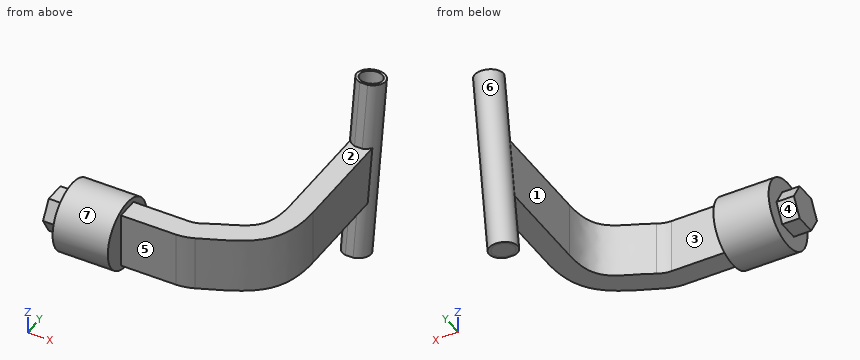
```python
from build123d import *

# Parameters (mm, degrees)
BOSS_EXTRUDE1_DEPTH      = 127
SKETCH2_R                = 78.74
BOSS_EXTRUDE2_DEPTH      = 127
BOSS_EXTRUDE3_DEPTH      = 40.132
BOSS_EXTRUDE4_DEPTH      = 12.7
BOSS_EXTRUDE4_DEPTH_BACK = 63.5
CUT_EXTRUDE4_DEPTH       = 719.599431417
SKETCH7_R                = 25.4
CUT_EXTRUDE5_DEPTH       = 304.8
BOSS_EXTRUDE5_DEPTH      = 50.8
SKETCH9_R                = 25.4
CUT_EXTRUDE6_DEPTH       = 706.793572447
SKETCH10_R               = 28.426883493
BOSS_EXTRUDE6_DEPTH      = 152.4


with BuildPart() as part:
    # Sketch1 → Boss-Extrude1 (new body)
    with BuildSketch(Plane.XY):
        with BuildLine():
            Line((0, 0), (127, 0))
            ThreePointArc((127, 0), (146.783062772, 2.389452828), (165.763803889, 8.456620544))
            add(Edge.make_bspline(
                [(165.763803889, 8.456620544), (215.95075425, 29.910933142), (293.749967936, 60.02479605), (329.40949352, 131.409080947), (329.40949352, 197.581697377)],
                knots=[0, 0, 0, 0, 0.489737158, 1, 1, 1, 1], degree=3))
            Line((329.40949352, 197.581697377), (329.40949352, 431.8))
            Line((329.40949352, 431.8), (278.60949352, 431.8))
            Line((278.60949352, 431.8), (278.60949352, 197.581697377))
            add(Edge.make_bspline(
                [(156.630652755, 58.428868346), (189.028044031, 76.295644753), (253.765909659, 94.018996051), (278.60949352, 141.969854777), (278.60949352, 197.581697377)],
                knots=[0, 0, 0, 0, 0.475110131, 1, 1, 1, 1], degree=3))
            ThreePointArc((156.630652755, 58.428868346), (142.298490244, 52.737817604), (127, 50.8))
            Line((127, 50.8), (0, 50.8))
            Line((0, 50.8), (0, 0))
        make_face()
    extrude(amount=BOSS_EXTRUDE1_DEPTH)

    # Sketch2 → Boss-Extrude2 (add)
    with BuildSketch(Plane.ZY):
        with Locations((63.5, 25.4)):
            Circle(SKETCH2_R)
    extrude(amount=BOSS_EXTRUDE2_DEPTH)

    # Sketch3 → Boss-Extrude3 (add)
    with BuildSketch(Plane.ZY.offset(127)):
        Polygon((63.5, 72.32702988), (22.86, 48.86351494), (22.86, 1.93648506), (63.5, -21.52702988), (104.14, 1.93648506), (104.14, 48.86351494), align=None)
    extrude(amount=BOSS_EXTRUDE3_DEPTH)

    # Sketch4 → Boss-Extrude4 (add, two sides: drawn at the far end of the back side and taken through both)
    with BuildSketch(Plane.ZY.offset(-278.60949352).offset(-BOSS_EXTRUDE4_DEPTH_BACK)):
        Polygon((-123.979561218, 390.165409655), (273.996216856, 449.279655757), (262.901002007, 523.976146929), (-135.074776066, 464.861900827), align=None)
    extrude(amount=BOSS_EXTRUDE4_DEPTH + BOSS_EXTRUDE4_DEPTH_BACK)

    # Sketch6 → Cut-Extrude4 (cut, through all)
    with BuildSketch(Plane(origin=(0, -9.595531889, -64.600151761), x_dir=(-1, 0, 0), z_dir=(0, -0.14692530866024317, -0.9891475894299558))):
        with BuildLine():
            Line((-342.10949352, 404.146909738), (-312.773498747, 404.146909738))
            ThreePointArc((-312.773498747, 404.146909738), (-322.933498747, 460.026909738), (-272.133498747, 434.626909738))
            ThreePointArc((-272.133498747, 434.626909738), (-278.483498747, 415.576909738), (-294.993498747, 404.146909738))
            Line((-294.993498747, 404.146909738), (-265.90949352, 404.146909738))
            Line((-265.90949352, 404.146909738), (-265.90949352, 479.662931787))
            Line((-265.90949352, 479.662931787), (-342.10949352, 479.662931787))
            Line((-342.10949352, 479.662931787), (-342.10949352, 404.146909738))
        make_face()
    extrude(amount=-CUT_EXTRUDE4_DEPTH, mode=Mode.SUBTRACT)

    # Sketch7 → Cut-Extrude5 (cut)
    with BuildSketch(Plane(origin=(0, -9.595531889, -64.600151761), x_dir=(-1, 0, 0), z_dir=(0, -0.14692530866024317, -0.9891475894299558))):
        with Locations(Location((-303.883498747, 434.626909738, 0), (0, 0, 90))):
            Circle(SKETCH7_R)
    extrude(amount=-CUT_EXTRUDE5_DEPTH, mode=Mode.SUBTRACT)

    # Sketch8 → Boss-Extrude5 (add)
    with BuildSketch(Plane.ZY.offset(-278.60949352)):
        Polygon((0, 400.877395826), (0, 426.277395826), (127, 445.141632467), (127, 419.741632467), align=None)
    extrude(amount=-BOSS_EXTRUDE5_DEPTH)

    # Sketch9 → Cut-Extrude6 (cut, through all)
    with BuildSketch(Plane(origin=(0, -9.595531889, -64.600151761), x_dir=(-1, 0, 0), z_dir=(0, -0.14692530866024317, -0.9891475894299558))):
        with Locations(Location((-303.883498747, 434.626909738, 0), (0, 0, 90))):
            Circle(SKETCH9_R)
    extrude(amount=-CUT_EXTRUDE6_DEPTH, mode=Mode.SUBTRACT)

    # Sketch10 → Boss-Extrude6 (add)
    with BuildSketch(Plane(origin=(0, -9.595531889, -64.600151761), x_dir=(-1, 0, 0), z_dir=(0, -0.14692530866024317, -0.9891475894299558))):
        with Locations((-303.883498747, 434.626909738)):
            Circle(SKETCH10_R)
    extrude(amount=-BOSS_EXTRUDE6_DEPTH)


solid = part.part
```
CAD build for the part. Positions are in the model's coordinates, mm. Face numbers are marked on the shaded views. A direction names the side the tool comes from. Round coordinates to 2 decimals unless told otherwise and drop trailing zeros. Order: outer loops, then holes, each group sorted by start corner. A loop starts at its lowest first (then second) coordinate and runs counter-clockwise, first axis right, second up.
Q1. Slice it at A-A (x = -38). Write the cut outline in (y, z).
Q2. Wall check: L1, parallel to X at y = 290.5, z = 94; L2, parallel to Z at x = 303, y = 320; L3, parallel to Y at x = 73.5, z = 80. Give the ranges that are in metal, low to high.
Q3. Slice it at B-B (x = 37). Write the cut outline in (y, z).
Q4. Two-plate mould, pull along Y, no slides. Class the marked faces 1, 2 and 3: pulls with the +Y half, pulls with the -Y half, needs draft (parallel to the pull), parting line crosses it, or undercut.
Q5. Which spindle directions (+Z, -Z, +X, -X, +Y, -Y) get a long thin tool onto all of the face, cutting with end or side? Do the marked faces 4, 5, 6 and 7. Say none if no direction does.
Q6. Drop flat-ended pins along their axis: pin 1 (20 mm diameter, centred on x = -141.5, y = 23.5, fed in from -Z); pin 2 (12 mm diameter, centred on x = 108, z = 104, fed in from -Y); pin 3 (1.5 mm diameter, centred on y = 399, z = 3, fed in from +X); pin 4 (12 mm diameter, centred on y = 143, z = -10, fed in from -X). Give the stop position or say it passes through.
Results below:
1. outline: circle Ø157.48 at (25.4, 63.5)
2. L1: x = 278.61 to 329.41
2. L2: z = 0 to 127
2. L3: y = 0 to 50.8
3. outline: (0, 0) - (50.8, 0) - (50.8, 127) - (0, 127) - close
4. face 1: undercut
4. face 2: needs draft
4. face 3: pulls with the +Y half
5. face 4: -Z, -X, +Y
5. face 5: +Z, -Z, +X, -Y
5. face 6: none
5. face 7: -X
6. pin 1: stops at z = 22.86
6. pin 2: stops at y = 0
6. pin 3: stops at x = 329.41
6. pin 4: passes through
